Geometry: final body of the model. Coordinates: model frame, mm. A direction names the side the tool comes from. Give positions to 0.01 mm unless a question says otherwise; leave off trailing zeros. Write each loop counter-clockwise with the first axis right and the second up, starting at its lowest first coordinate (ties: lowest second). Pieces come first, ordered by that corner, then holes. Notation, with made-up numbers: (7.25, 82.5) -> (35.25, 82.5) arc R6 cw to (35.25, 86.5) -> close; hole circle Ø6 at (-36, 2.25). An arc over 180 degrees is marked (long way). Answer as a JSON object with one key per item and string values.
from build123d import *

# Parameters (mm, degrees)
F0_W           = 76.2
F0_H           = 76.2
F1_DEPTH       = 12.7
F3_D           = 3.175
F3_CBORE_D     = 6.35
F3_CBORE_DEPTH = 6.35


with BuildPart() as f1:
    # F0 (on Front) → F1 (new body)
    with BuildSketch(Plane.XZ):
        Rectangle(F0_W, F0_H)
    extrude(amount=F1_DEPTH)

    # F3 (through all)
    with Locations(Plane.XZ.offset(12.7)):
        with Locations((-24.05159, 22.108026), (22.917846, 22.108026), (22.917846, -25.509261), (-24.05159, -25.509261)):
            CounterBoreHole(F3_D / 2, F3_CBORE_D / 2, F3_CBORE_DEPTH)


solid = f1.part
Q1. Cut plane A-A (x = -23.5). Return the cut outline in (y, z).
Values:
{"outline": "(-12.7, -38.1) -> (0, -38.1) -> (0, -27) -> (-6.35, -27) -> (-6.35, -28.64) -> (-12.7, -28.64) -> close; (-12.7, -22.38) -> (-6.35, -22.38) -> (-6.35, -24.02) -> (0, -24.02) -> (0, 20.62) -> (-6.35, 20.62) -> (-6.35, 18.98) -> (-12.7, 18.98) -> close; (-12.7, 25.23) -> (-6.35, 25.23) -> (-6.35, 23.6) -> (0, 23.6) -> (0, 38.1) -> (-12.7, 38.1) -> close"}
Q2. Mould query, pull axis X, two halves, no side actions, for faces 3 (the flat face through (21, -6.35, 21)), 4 (the flat face through (-1, 0, 1)), 5 (the flat face through (38.1, -6, -1)), 6 (the cylindrical face through (-24.905, -3.131, 23.447)). Classes: pulls with the +X half, pulls with the -X half, needs draft (parallel to the pull), parting line crosses it, or undercut.
Values:
{"face 3": "undercut", "face 4": "needs draft", "face 5": "pulls with the +X half", "face 6": "undercut"}
Q3. First-contact query: P1, Ø5, axis at x = -24.05, z = -25.51, coming from the -Y side. Flat tip, straight axial feed; report the tip coordinate or a pass-through.
Values:
{"P1": "y = -6.35"}
Q4. Material intervals for L1, parallel to Z at x = 23, y = -2.25; L2, parallel to Y at x = 20, z = -25.5, sorted ascending. Write a range as from..to.
Values:
{"L1": "-38.1..-27.09, -23.92..20.52, 23.69..38.1", "L2": "-6.35..0"}
Q5. Set-up query: faces 1 (the cylindrical face through (-24.905, -3.131, -24.171)), 2 (the flat face through (21, -6.35, -26)). Return all of +Z, -Z, +X, -X, +Y, -Y with unobstructed straight access to the full face (end or side cutting, diameter ignored); none if empty.
Values:
{"face 1": "+Y, -Y", "face 2": "-Y"}
Q6. Cut plane B-B (y = -9.25). Return the cut outline in (x, z) (3 decimals), and give its area (3 significant figures).
Values:
{"outline": "(-38.1, -38.1) -> (38.1, -38.1) -> (38.1, 38.1) -> (-38.1, 38.1) -> close; hole circle Ø6.35 at (-24.052, -25.509); hole circle Ø6.35 at (-24.052, 22.108); hole circle Ø6.35 at (22.918, -25.509); hole circle Ø6.35 at (22.918, 22.108)", "area": "5,680 mm²"}
